Input: part model. Units: mm. Frame: model coordinates. A direction names the side the tool comes from. Round coordinates to 2 decimals unless told otherwise and drop trailing zeros. Write each loop counter-clockwise with the first axis right and the second up, starting at its lowest first coordinate (ties: lowest second). Pieces come first, ordered by that corner, then holes. Notation, with made-up numbers: (-33, -35) -> (3, -35) arc R35 cw to (3, -3) -> close; hole circle Ø7 at (-18.75, 4). An arc over 180 degrees is marked (long way). Use CSV: the item, a comma, the result in double quotes.
```python
from build123d import *

# Parameters (mm, degrees)
BOSS_EXTRUDE1_DEPTH = 5
CUT_EXTRUDE1_DEPTH  = 5
SKETCH4_R           = 2
CUT_EXTRUDE2_DEPTH  = 5


with BuildPart() as part:
    # Sketch1 → Boss-Extrude1 (new body)
    with BuildSketch(Plane.XY):
        Polygon((10, -30), (47.5, -30), (47.5, 30), (-47.5, 30), (-47.5, -30), (-10, -30), (-10, -34.9), (10, -34.9), align=None)
    extrude(amount=BOSS_EXTRUDE1_DEPTH)

    # Sketch3 → Cut-Extrude1 (cut)
    with BuildSketch(Plane.XY.offset(5)):
        Polygon((-33.1, -27), (-33.1, -30), (-37.5, -30), (-37.5, -27), (-39, -27), (-39, -23.6), (-37.5, -23.6), (-37.5, -9.8), (-33.1, -9.8), (-33.1, -23.6), (-31.6, -23.6), (-31.6, -27), align=None)
        Polygon((37.5, -30), (37.5, -27), (39, -27), (39, -23.6), (37.5, -23.6), (37.5, -9.8), (33.1, -9.8), (33.1, -23.6), (31.6, -23.6), (31.6, -27), (33.1, -27), (33.1, -30), align=None)
        Polygon((33.1, 27), (33.1, 30), (37.5, 30), (37.5, 27), (39, 27), (39, 23.6), (37.5, 23.6), (37.5, 9.8), (33.1, 9.8), (33.1, 23.6), (31.6, 23.6), (31.6, 27), align=None)
        Polygon((-37.5, 30), (-37.5, 27), (-39, 27), (-39, 23.6), (-37.5, 23.6), (-37.5, 9.8), (-33.1, 9.8), (-33.1, 23.6), (-31.6, 23.6), (-31.6, 27), (-33.1, 27), (-33.1, 30), align=None)
    extrude(amount=-CUT_EXTRUDE1_DEPTH, mode=Mode.SUBTRACT)

    # Sketch4 → Cut-Extrude2 (cut)
    with BuildSketch(Plane.XY.offset(5)):
        with Locations((10, -9.7)):
            Circle(SKETCH4_R)
    extrude(amount=-CUT_EXTRUDE2_DEPTH, mode=Mode.SUBTRACT)


solid = part.part
```
Item 1: Line query: line 1 (X direction, y = -18.5, z = 0.7); line 2 (Y direction, x = 32, z = 4); line 3 (Y direction, x = -34, z = 2.85). Output: solid intervals per line, ascending.
Worked answers:
line 1,"x = -47.5 to -37.5, -33.1 to 33.1, 37.5 to 47.5"
line 2,"y = -30 to -27, -23.6 to 23.6, 27 to 30"
line 3,"y = -9.8 to 9.8"
Item 2: First-contact query: pin 1 Ø1.2 at (x, z) = (-32, 1.5) entering from -Y. Flat tip, straight axial feed; report the tip coordinate or a pass-through.
Worked answers:
pin 1,"stops at y = -30"
Item 3: Pull-direction query (X, two-part tool) for faces 5 (the face through (42, -30, 2)), 6 (the face through (-35, -9.8, 3)), 7 (the face through (-47.5, 0, 2)); classes: +X half, -X half, draft (parallel to the pull), parting line (faces both ways), or undercut.
Worked answers:
face 5,"draft"
face 6,"undercut"
face 7,"-X half"
Item 4: Section query B-B on y = -31. Return the cut outline in (x, z).
Worked answers:
outline,"(-10, 0) -> (10, 0) -> (10, 5) -> (-10, 5) -> close"
Item 5: Section query A-A on y = 16.5. Return the cut outline in (x, z), plus the area to 3 significant figures.
Worked answers:
outline,"(-47.5, 0) -> (-37.5, 0) -> (-37.5, 5) -> (-47.5, 5) -> close; (-33.1, 0) -> (33.1, 0) -> (33.1, 5) -> (-33.1, 5) -> close; (37.5, 0) -> (47.5, 0) -> (47.5, 5) -> (37.5, 5) -> close"
area,"431 mm²"
Item 6: Set-up query: faces 1 (the face through (-22, -30, 2)), 2 (the face through (-37.5, -29, 3)), 3 (the face through (37.5, 29, 3)), 4 (the face through (31.6, 25, 3)). Return all of +Z, -Z, +X, -X, +Y, -Y with unobstructed straight access to the full face (end or side cutting, diameter ignored); none if empty.
Worked answers:
face 1,"+Z, -Z, -X, -Y"
face 2,"+Z, -Z, -Y"
face 3,"+Z, -Z, +Y"
face 4,"+Z, -Z"
